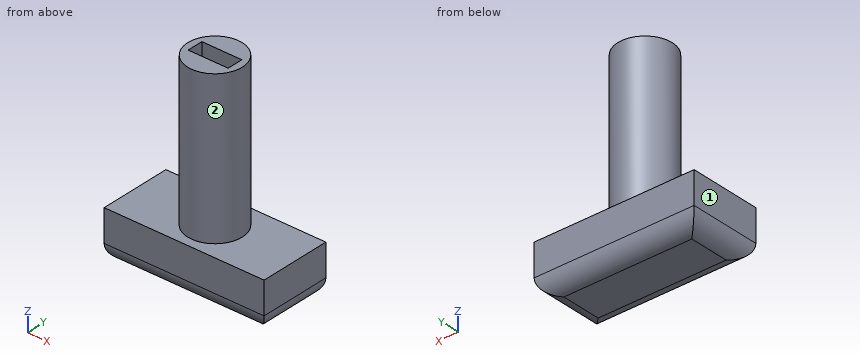
```python
from build123d import *

# Parameters (mm, degrees)
F0_R     = 4.318
F0_W     = 6.35
F0_H     = 2.54
F1_DEPTH = 24.13
F2_W     = 25.4
F2_H     = 11.43
F2_R     = 4.318
F2_W_2   = 6.35
F2_H_2   = 2.54
F3_DEPTH = 7.62
F4_R     = 2.54


with BuildPart() as f1:
    # F0 (on Top) → F1 (new body)
    with BuildSketch(Plane.XY):
        Circle(F0_R)
        Rectangle(F0_W, F0_H, mode=Mode.SUBTRACT)
    extrude(amount=F1_DEPTH)

    # F2 (on face) → F3 (join)
    with BuildSketch(Plane(origin=(0, 0, 0), x_dir=(1, 0, 0), z_dir=(0, 0, -1))):
        Rectangle(F2_W, F2_H)
        Circle(F2_R, mode=Mode.SUBTRACT)
        Circle(F2_R)
        Rectangle(F2_W_2, F2_H_2, mode=Mode.SUBTRACT)
        Rectangle(F2_W_2, F2_H_2)
    extrude(amount=F3_DEPTH)

    # F4
    f4_edges = [f1.edges().sort_by_distance(p)[0] for p in [
        (12.7, 0, -7.62),
        (0, -5.715, -7.62),
        (-12.7, 0, -7.62),
        (0, 5.715, -7.62),
    ]]
    fillet(f4_edges, radius=F4_R)


solid = f1.part
```
CAD build for the part. Positions are in the model's coordinates, mm. Face numbers are marked on the shaded views. A direction names the side the tool comes from. Coordinates: 2 decimals unless noted, no trailing zeros. Order: outer loops, then holes, each group sorted by start corner. A loop starts at its lowest first (then second) coordinate and runs counter-clockwise, first axis right, second up. Notation, with made-up numbers: (39.25, -26.75) - (91.25, -26.75) arc R17 ccw to (91.25, -21.75) - close; hole circle Ø7 at (-7.5, 79.5). An arc over 180 degrees is marked (long way). Use a Markdown table: item, result. Add a question column.
(1) Drill centre lines: line 1 along Z through (x, y) = (7.25, 1.25); line 2 along Y through (x, z) = (-1.5, 22.5); line 3 along X through (y, z) = (-0.5, 4.5) (3 decimals). Where is each one in solid material? Low to high. Write a range as [from, to].
(2) Saw through at A-A (z = 14). Give the cut face in (x, y) (3 decimals), then the cut area to 3 significant figures.
(3) Saw through at C-C (x = 0). Give the cut face in (y, z) (3 decimals).
(4) Flat gauge pins, fed straight in: pin 1 (2 mm diameter, centred on y = 2, z = 4, fed in from -X); pin 2 (7 mm diameter, centred on x = -1, z = 15.5, fed in from +Y); pin 3 (4 mm diameter, centred on y = 2, z = 14.5, fed in from +X). Where does each tip first touch, or does it go through?
(5) Which spindle directions (+Z, -Z, +X, -X, +Y, -Y) get a long thin tool onto all of the face, cutting with end or side? Do the marked faces 1 and 2. Say none if no direction does.
(6) Saw through at B-B (y = 0). Give the cut face in (x, z) (3 decimals), then the cut area to 3 significant figures.
(7) Saw through at D-D (y = 3.75). Give the cut face in (x, z) (3 decimals), then the cut area to 3 significant figures.
Solved:
| question | item | result |
|---|---|---|
| 1 | line 1 | z = [-7.62, 0] |
| 1 | line 2 | y = [-4.05, -1.27], [1.27, 4.05] |
| 1 | line 3 | x = [-4.289, -3.175], [3.175, 4.289] |
| 2 | outline | circle Ø8.636 at (0, 0); hole (-3.175, -1.27) - (3.175, -1.27) - (3.175, 1.27) - (-3.175, 1.27) - close |
| 2 | area | 42.4 mm² |
| 3 | outline | (-5.715, -5.08) arc R2.54 ccw to (-3.175, -7.62) - (3.175, -7.62) arc R2.54 ccw to (5.715, -5.08) - (5.715, 0) - (4.318, 0) - (4.318, 24.13) - (1.27, 24.13) - (1.27, 0) - (-1.27, 0) - (-1.27, 24.13) - (-4.318, 24.13) - (-4.318, 0) - (-5.715, 0) - close |
| 4 | pin 1 | stops at x = -4.2 |
| 4 | pin 2 | stops at y = 4.32 |
| 4 | pin 3 | stops at x = 4.32 |
| 5 | face 1 | +Z, -Z, -X, +Y, -Y |
| 5 | face 2 | +Z |
| 6 | outline | (-12.7, -5.08) arc R2.54 ccw to (-10.16, -7.62) - (10.16, -7.62) arc R2.54 ccw to (12.7, -5.08) - (12.7, 0) - (4.318, 0) - (4.318, 24.13) - (3.175, 24.13) - (3.175, 0) - (-3.175, 0) - (-3.175, 24.13) - (-4.318, 24.13) - (-4.318, 0) - (-12.7, 0) - close |
| 6 | area | 246 mm² |
| 7 | outline | (-12.7, -5.08) arc R2.54 ccw to (-10.735, -7.554) - (10.735, -7.554) arc R2.54 ccw to (12.7, -5.08) - (12.7, 0) - (2.141, 0) - (2.141, 24.13) - (-2.141, 24.13) - (-2.141, 0) - (-12.7, 0) - close |
| 7 | area | 293 mm² |
